Check sheet for the drawn part. Datum: minimum x, y, z corner. Units: mm. A direction names the side the tool comes from. Coordinates: 2 decimals unless noted, no trailing zeros. Write each loop counter-clockwise with the first axis right and the second up, starting at its lowest first coordinate (ties: lowest second). Pieces come first, ordered by that corner, then holes. Notation, with made-up numbers: M 74,73.5 L 119,73.5 A11 cw 119,88.5 Z; hole C -10,-26.5 d5. An arc over 180 degrees is marked long. Answer as CSV lines item,"result".
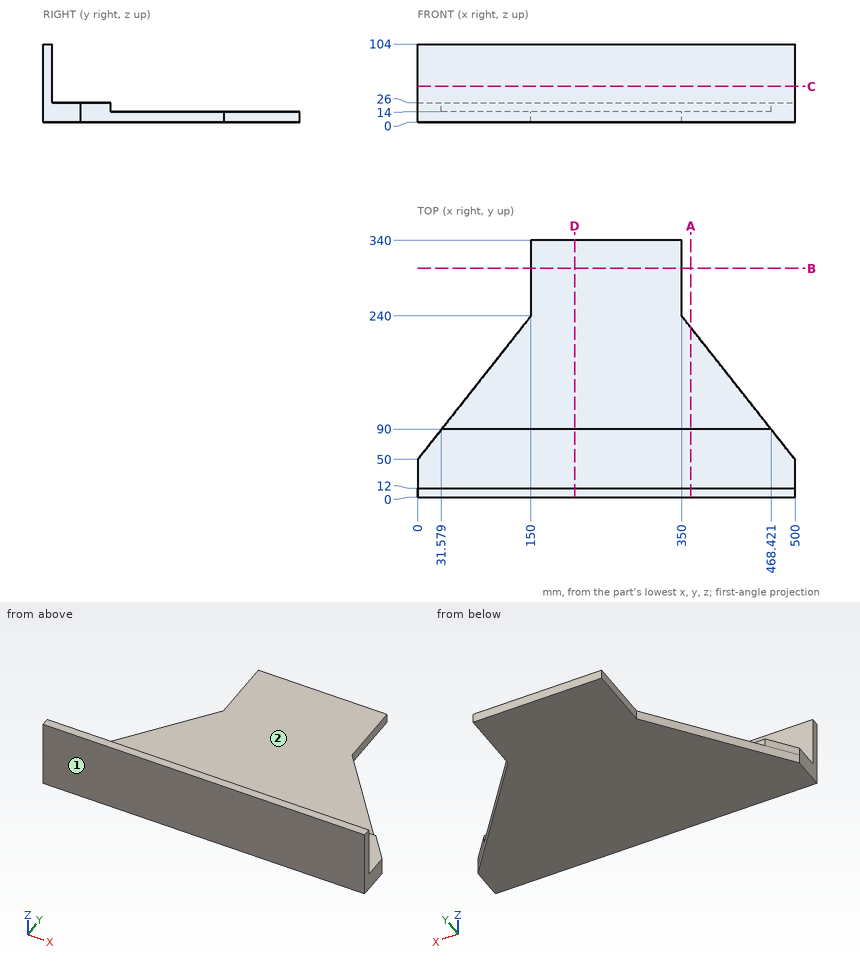
1) Thickness scan on line 1 along Z through (x, y) = (169, 144); line 2 along Y through (x, z) = (152, 63); line 3 along Y through (x, z) = (86.5, 22). Record the ranges inside material, lowest first.
Answer key:
line 1,"z = 0 to 14"
line 2,"y = 0 to 12"
line 3,"y = 0 to 90"
2) Depth check by flat-ended pin: P1, Ø5, axis at x = 129, z = 31, coming from the +Y side; P2, Ø7, axis at y = 265.5, z = 3.5, coming from the +X side; P3, Ø10, axis at x = 97.5, z = 28, coming from the +Y side. Enter the tip coordinate at first touch or a pass-through.
Answer key:
P1,"stops at y = 12"
P2,"stops at x = 350"
P3,"stops at y = 90"
3) Section check A-A, the plane x = 362. Record the boundary of the cut face in (y, z).
Answer key:
outline,"M 0,0 L 224.8,0 L 224.8,14 L 90,14 L 90,26 L 12,26 L 12,104 L 0,104 Z"
4) Section check C-C, the plane z = 48. Record the boundary of the cut face in (x, y), plus the area to 3 significant figures.
Answer key:
outline,"M 0,0 L 500,0 L 500,12 L 0,12 Z"
area,"6,000 mm2"
5) Section check D-D, the plane x = 208. Record the boundary of the cut face in (y, z).
Answer key:
outline,"M 0,0 L 340,0 L 340,14 L 90,14 L 90,26 L 12,26 L 12,104 L 0,104 Z"
6) Tool access check on the marked faces 1 and 2. Record the directions out of +Z, -Z, +X, -X, +Y, -Y that give a thin tool (end or side, any length) a straight path to the whole face; none if there is none.
Answer key:
face 1,"+Z, -Z, +X, -X, -Y"
face 2,"+Z, +X, -X, +Y"
7) Section check B-B, the plane y = 303. Record the boundary of the cut face in (x, z).
Answer key:
outline,"M 150,0 L 350,0 L 350,14 L 150,14 Z"
